Input: part model. Units: mm. Frame: model coordinates. Give positions to 0.01 mm unless a question says otherwise; leave off trailing zeros. Write each loop counter-clockwise with the first axis right and the second up, starting at its lowest first coordinate (ties: lowest second). Pieces come first, ordered by that corner, then holes.
```python
from build123d import *

# Parameters (mm, degrees)
SKETCH_1_W          = 25.05955055
SKETCH_1_H          = 183.842173556
EXTRUDE_1_DEPTH     = 5
SKETCH_2_R          = 10
CUT_EXTRUDE_1_DEPTH = 5
FILLET_1_R          = 12.5


with BuildPart() as part:
    # 草图1 → 凸台-拉伸1 (new body)
    with BuildSketch(Plane.XY):
        Rectangle(SKETCH_1_W, SKETCH_1_H)
    extrude(amount=EXTRUDE_1_DEPTH)

    # 草图2 → 切除-拉伸1 (cut)
    with BuildSketch(Plane(origin=(0, 0, 0), x_dir=(-1, 0, 0), z_dir=(0, 0, -1))):
        with Locations((0, 75.312469171)):
            Circle(SKETCH_2_R)
        with Locations((0, -74.807016358)):
            Circle(SKETCH_2_R)
    extrude(amount=-CUT_EXTRUDE_1_DEPTH, mode=Mode.SUBTRACT)

    # 圆角1
    fillet_1_edges = [part.edges().sort_by_distance(p)[0] for p in [
        (-12.529775275, 91.921086778, 2.5),
        (12.529775275, 91.921086778, 2.5),
        (12.529775275, -91.921086778, 2.5),
        (-12.529775275, -91.921086778, 2.5),
    ]]
    fillet(fillet_1_edges, radius=FILLET_1_R)


solid = part.part
```
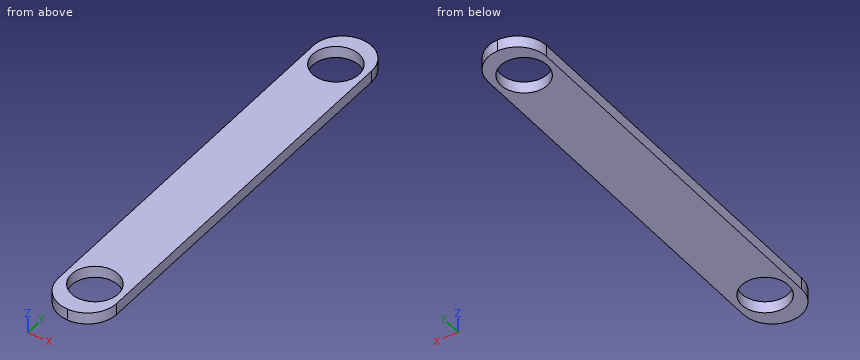
Q1. Section C-C, the plane z = 3.9. Return the cut outline in (x, y), then the cut area to 3 significant figures.
Q2. Section A-A, the plane y = 68.5. Return the cut outline in (x, z), then the cut area to 3 significant figures.
Q3. Section B-B, the plane x = 8. Return the cut outline in (y, z).
Q4. Material intervals for line 1 along Y through (x, z) = (0, 3.5); line 2 along Y through (x, z) = (-3.75, 0.9); line 3 along X through (y, z) = (71, 1.75), sorted ascending.
Q5. Pin query (flat end, axial travel): pin 1 (8 mm diameter, centred on x = 3.5, y = 60, fed in from -Z). Return the tip coordinate at first contact, or that it passes through.
Solutions:
1. outline: (-12.53, -79.42) arc R12.5 ccw to (-0.03, -91.92) - (0.03, -91.92) arc R12.5 ccw to (12.53, -79.42) - (12.53, 79.42) arc R12.5 ccw to (0.03, 91.92) - (-0.03, 91.92) arc R12.5 ccw to (-12.53, 79.42) - close; hole circle Ø20 at (0, -74.81); hole circle Ø20 at (0, 75.31)
1. area: 3,840 mm2
2. outline: (-12.53, 0) - (-7.32, 0) - (-7.32, 5) - (-12.53, 5) - close; (7.32, 0) - (12.53, 0) - (12.53, 5) - (7.32, 5) - close
2. area: 52.1 mm2
3. outline: (-89.05, 0) - (-80.81, 0) - (-80.81, 5) - (-89.05, 5) - close; (-68.81, 0) - (69.31, 0) - (69.31, 5) - (-68.81, 5) - close; (81.31, 0) - (89.05, 0) - (89.05, 5) - (81.31, 5) - close
4. line 1: y = -91.92 to -84.81, -64.81 to 65.31, 85.31 to 91.92
4. line 2: y = -91.35 to -84.08, -65.54 to 66.04, 84.58 to 91.35
4. line 3: x = -12.53 to -9.02, 9.02 to 12.53
5. pin 1: stops at z = 0
